Check sheet for the modelled part. Datum: model origin and axes. Units: mm. A direction names the side the tool comes from. Round coordinates to 2 decimals unless told otherwise and drop trailing zeros. Loops run counter-clockwise (first coordinate to the right, second up) from the corner with the lowest first, then second, coordinate; pieces in that order, holes last. Notation, with made-up numbers: M -33.75,27 L 17.25,27 A17 ccw 17.25,59 Z; hole C 22,0.5 d9. An arc over 180 degrees is marked long. Write item = value, one per line. Start each with the question number.
(1) Go/stop test with flat-tipped pins: P1, Ø6, axis at x = 8, z = 56.5, coming from the -Y side; P2, Ø6, axis at y = -9.5, z = 56, coming from the +X side; P3, Ø6.5, axis at y = 0.5, z = 14.5, coming from the +X side. Record where each tip stops, or that it passes through.
(2) Cross-section at C-C on z = 45. Record the boundary of the cut face in (x, y).
(3) Scan lines: L1, parallel to Z at x = 3.75, y = 0 (3 decimals); L2, parallel to Z at x = 7.25, y = 0.75; L3, parallel to X at y = -4.5, z = 80. Record each from-to range of solid material in increasing order. Write a range as from..to.
(4) Mould release check, pull along Y, two halves, no side actions. Record for faces 4 (the face through (5.83, -11.21, 76.72)), 5 (the face through (9, 0, 25.4)), 6 (the face through (-0.089, -1.707, 9.027)): pulls with the +Y half, pulls with the -Y half, needs draft (parallel to the pull), parting line crosses it, or undercut.
(5) Cross-section at D-D on y = -7.5. Record the boundary of the cut face in (x, z).
(6) Set-up check for faces 1 (the face through (0, 0, 0)), 2 (the face through (6.35, 0, 13)), 3 (the face through (-6.35, 0, 13)): record each of +Z, -Z, +X, -X, +Y, -Y from which the full face is reachable in a straight line by a thin tool's end or side.
from build123d import *

# Parameters (mm, degrees)
F0_R     = 12.6365
F1_DEPTH = 127
F2_W     = 13.516908
F2_H     = 36.040129
F3_DEPTH = 12.7
F4_R     = 3.175
F5_DEPTH = 25.4


with BuildPart() as f1:
    # F0 (on Top) → F1 (new body)
    with BuildSketch(Plane.XY):
        Circle(F0_R)
    extrude(amount=F1_DEPTH)

    # F2 (on Front) → F3 (cut, symmetric)
    with BuildSketch(Plane.XZ):
        with Locations((-13.108454, 7.379935)):
            Rectangle(F2_W, F2_H)
        with Locations((13.108454, 7.379935)):
            Rectangle(F2_W, F2_H)
    extrude(amount=F3_DEPTH, both=True, mode=Mode.SUBTRACT)

    # F4 (on face) → F5 (cut)
    with BuildSketch(Plane(origin=(-6.35, 0, 0), x_dir=(0, -1, 0), z_dir=(-1, 0, 0))):
        with Locations((0, 6.35)):
            Circle(F4_R)
    extrude(amount=-F5_DEPTH, mode=Mode.SUBTRACT)


solid = f1.part
Result:
q1.P1 = -11.61
q1.P2 = 10.84
q1.P3 = 6.35
q2.outline = C 0,0 d25.27
q3.L1 = 0..3.175, 9.525..127
q3.L2 = 25.4..127
q3.L3 = -11.81..11.81
q4.face_4 = parting line crosses it
q4.face_5 = needs draft
q4.face_6 = undercut
q5.outline = M -10.17,25.4 L -6.35,25.4 L -6.35,0 L 6.35,0 L 6.35,25.4 L 10.17,25.4 L 10.17,127 L -10.17,127 Z
q6.face_1 = -Z, +X, -X, +Y, -Y
q6.face_2 = -Z, +X, +Y, -Y
q6.face_3 = -Z, -X, +Y, -Y
